Geometry check sheet. Reference: drawing and pictorial views, mm from the part's lowest x, y, z. A direction names the side the tool comes from. Coordinates: 2 decimals unless noted, no trailing zeros. Loops run counter-clockwise (first coordinate to the right, second up) from the corner with the lowest first, then second, coordinate; pieces in that order, holes last. Notation, with made-up numbers: (66.5, 64.25) -> (78.5, 64.25) arc R12 ccw to (78.5, 76.25) -> close; hole circle Ø8 at (-27.5, -16). An arc over 180 degrees is marked (long way). Use one line per item in the form item = value.
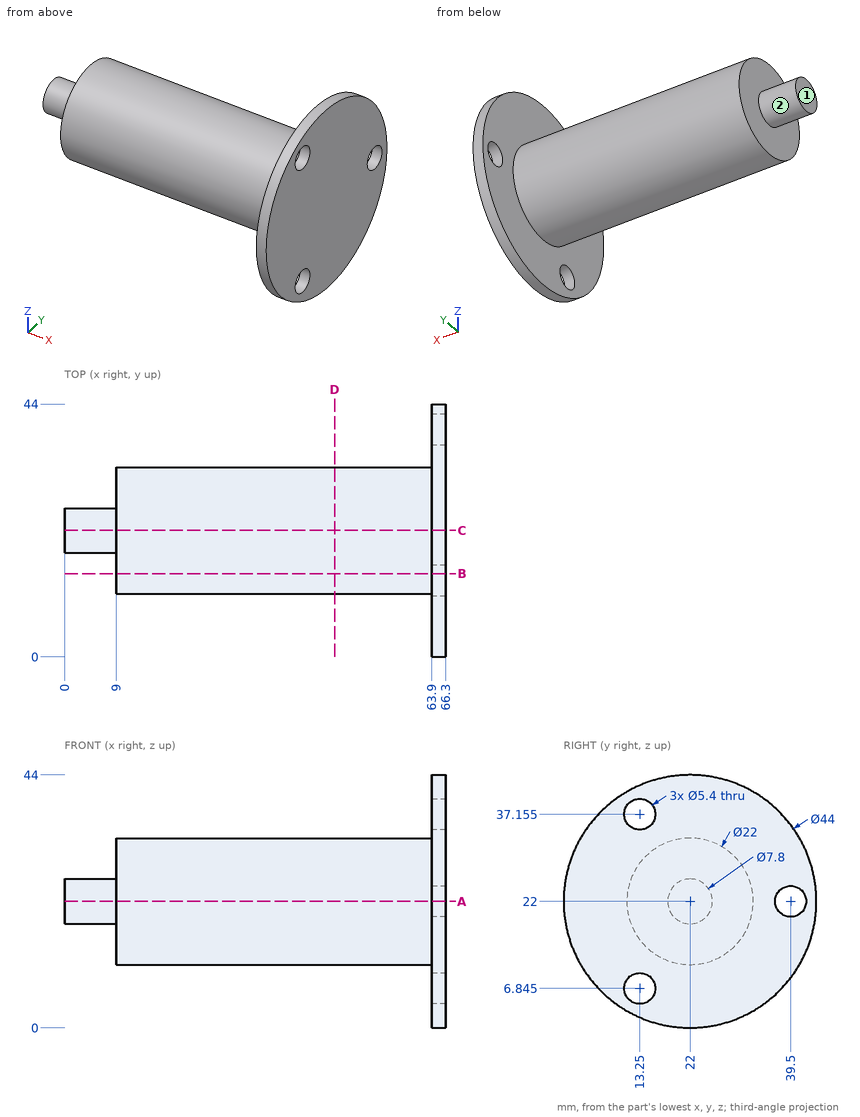
(1) Go/stop test with flat-tipped pins: P1, Ø10, axis at x = 16.5, z = 14, coming from the +Y side; P2, Ø5, axis at x = 21.5, z = 31, coming from the -Y side (1 decimal); P3, Ø12, axis at y = 35.5, z = 37.5, coming from the -X side. Record where each tip stops, or that it passes through.
Established:
P1 = 32.58
P2 = 13.1
P3 = 63.9
(2) Section check C-C, the plane y = 22. Record the boundary of the cut face in (x, z), plus the area to 3 significant figures.
Established:
outline = (0, 18.1) -> (9, 18.1) -> (9, 11) -> (63.9, 11) -> (63.9, 0) -> (66.3, 0) -> (66.3, 44) -> (63.9, 44) -> (63.9, 33) -> (9, 33) -> (9, 25.9) -> (0, 25.9) -> close
area = 1,380 mm²
(3) Tool access check on the marked faces 1 and 2. Record the directions out of +Z, -Z, +X, -X, +Y, -Y that give a thin tool (end or side, any length) a straight path to the whole face; none if there is none.
Established:
face_1 = +Z, -Z, -X, +Y, -Y
face_2 = -X
(4) Section check A-A, the plane z = 22. Record the boundary of the cut face in (x, y), plus the area to 3 significant figures.
Established:
outline = (0, 18.1) -> (9, 18.1) -> (9, 11) -> (63.9, 11) -> (63.9, 0) -> (66.3, 0) -> (66.3, 36.8) -> (63.9, 36.8) -> (63.9, 33) -> (9, 33) -> (9, 25.9) -> (0, 25.9) -> close; (63.9, 42.2) -> (66.3, 42.2) -> (66.3, 44) -> (63.9, 44) -> close
area = 1,370 mm²
(5) Scan lines: line 1 along Y through (x, z) = (65, 22); line 2 along X through (y, z) = (17, 38); line 3 along X through (y, z) = (23, 31.5). Record each from-to range of solid material in increasing order.
Established:
line_1 = 0 to 36.8, 42.2 to 44
line_2 = 63.9 to 66.3
line_3 = 9 to 66.3
(6) Section check D-D, the plane x = 47. Record the boundary of the cut face in (y, z), plus the area to 3 significant figures.
Established:
outline = circle Ø22 at (22, 22)
area = 380 mm²
(7) Section check B-B, the plane y = 14.5. Record the boundary of the cut face in (x, z).
Established:
outline = (9, 13.95) -> (63.9, 13.95) -> (63.9, 9.24) -> (66.3, 9.24) -> (66.3, 34.76) -> (63.9, 34.76) -> (63.9, 30.05) -> (9, 30.05) -> close; (63.9, 1.32) -> (66.3, 1.32) -> (66.3, 4.45) -> (63.9, 4.45) -> close; (63.9, 39.55) -> (66.3, 39.55) -> (66.3, 42.68) -> (63.9, 42.68) -> close
